For this review, use the dimensioned drawing (mm, ordinates from the lowest corner) and the shaded views. A direction names the side the tool comes from. Give positions to 0.01 mm unless a question says otherwise; leave off trailing zeros. Order: outer loops, then holes, each group sorted by start corner. A loop starts at its lowest first (then second) coordinate and runs counter-clockwise, first axis right, second up.
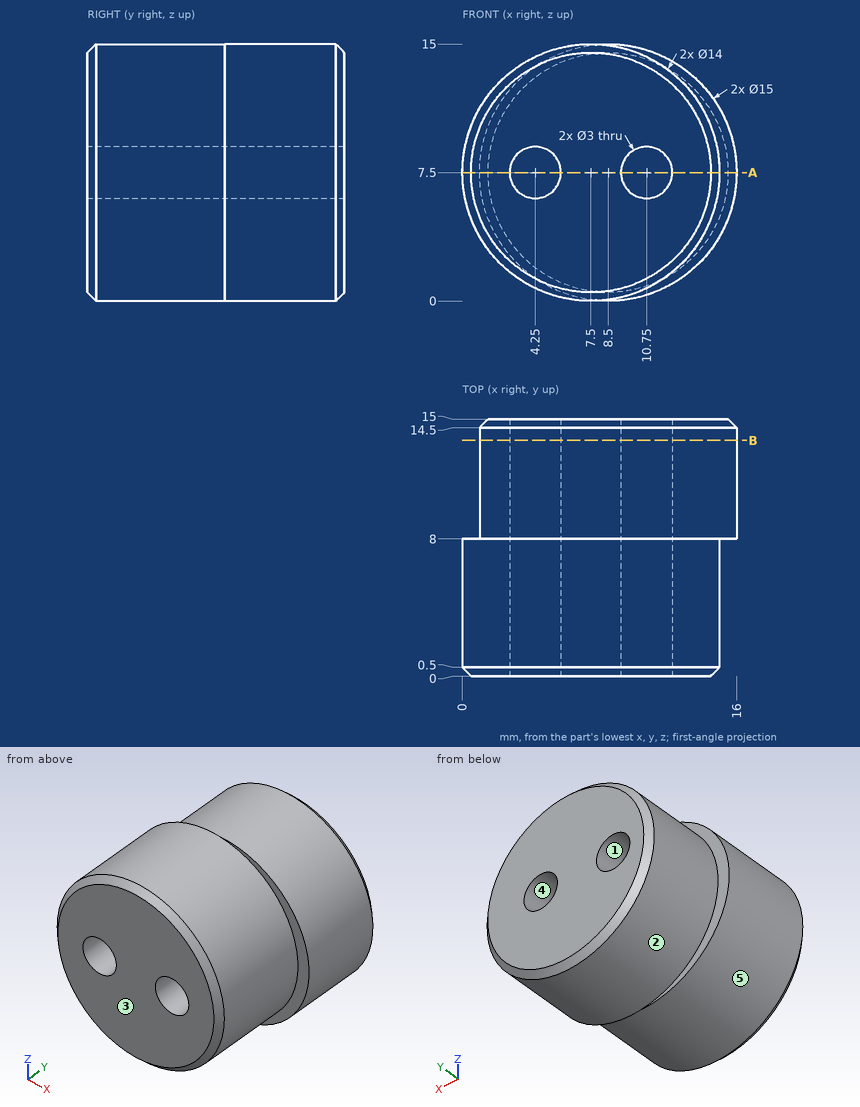
1. Draft analysis for pull direction X (two halves, no side actions). For the marked faces 3, 4 and 5, state which applies: pulls with the +X half, pulls with the -X half, needs draft (parallel to the pull), parting line crosses it, or undercut.
Recorded:
face 3: needs draft
face 4: undercut
face 5: parting line crosses it
2. For pin 1 (1 mm diameter, centred on x = 10.5, z = 2.5, fed in from -Y); pin 2 (1.5 mm diameter, centred on y = 12.5, z = 13, fed in from -X); pin 3 (4 mm diameter, centred on x = 11, y = 8.5, fed in from +Z); pin 4 (3 mm diameter, centred on x = 14, y = 11, fed in from +Z), all flat-tipped, find the tip position at first contact; note any pin that passes through.
Recorded:
pin 1: stops at y = 0
pin 2: stops at x = 2.7
pin 3: stops at z = 14.98
pin 4: stops at z = 13.84
3. Take a section at A-A (z = 7.5). State the section outline as (x, y) points.
Recorded:
outline: (0, 0.5) - (0.5, 0) - (2.75, 0) - (2.75, 15) - (1.5, 15) - (1, 14.5) - (1, 8) - (0, 8) - close; (5.75, 0) - (9.25, 0) - (9.25, 15) - (5.75, 15) - close; (12.25, 0) - (14.5, 0) - (15, 0.5) - (15, 8) - (16, 8) - (16, 14.5) - (15.5, 15) - (12.25, 15) - close
4. For line 1 along X through (y, z) = (7, 7.5); line 2 along Z through (x, y) = (12, 3); line 3 along Y through (x, z) = (1.5, 4), list the stretches that pass through material, from the lowest coordinate up.
Recorded:
line 1: x = 0 to 2.75, 5.75 to 9.25, 12.25 to 15
line 2: z = 1.5 to 6.67, 8.33 to 13.5
line 3: y = 0 to 8
5. Machinability: for the marked faces 1 and 2, which of the approach directions +Z, -Z, +X, -X, +Y, -Y give a long, thin tool a straight path to every point of the face, cutting with its end or side? Answer none if there is none.
Recorded:
face 1: +Y, -Y
face 2: +Y
6. Take a section at B-B (y = 13.75). State the section outline as (x, z) points.
Recorded:
outline: circle Ø15 at (8.5, 7.5); hole circle Ø3 at (4.25, 7.5); hole circle Ø3 at (10.75, 7.5)
